Design review of the part built by this model. Coordinates are the model's own, in mm. A direction names the side the tool comes from. Give positions to 0.01 mm unless a question says otherwise; leave off trailing zeros. Write each loop counter-clockwise with the first axis right and the second up, starting at its lowest first coordinate (ties: lowest second). Pieces come first, ordered by that corner, then holes. Notation, with made-up numbers: M 79,47.5 L 138,47.5 A29 cw 138,77.5 Z; hole C 87,-15 d9. An arc over 180 degrees is marked long. Use one line per item in the form item = value. Start each with the question number.
from build123d import *

# Parameters (mm, degrees)
SKETCH1_R           = 215
PLATE_DEPTH         = 20
SKETCH2_R           = 204
SKETCH2_R_2         = 144
COMB_GROOVE_DEPTH   = 4
SKETCH3_R           = 2.75
ROD_HOLES_DEPTH     = 20
SKETCH4_R           = 5
NUT_POCKETS_DEPTH   = 6
SKETCH5_W           = 40
SKETCH5_H           = 30
PD_POCKET_DEPTH     = 8
SKETCH6_W           = 60
SKETCH6_H           = 12
CABLE_CHANNEL_DEPTH = 8


with BuildPart() as part:
    # Sketch1 → Plate (new body)
    with BuildSketch(Plane.XY):
        Circle(SKETCH1_R)
    extrude(amount=PLATE_DEPTH)

    # Sketch2 → Comb_groove (cut)
    with BuildSketch(Plane.XY.offset(16)):
        Circle(SKETCH2_R)
        Circle(SKETCH2_R_2, mode=Mode.SUBTRACT)
    extrude(amount=COMB_GROOVE_DEPTH, mode=Mode.SUBTRACT)

    # Sketch3 → Rod_holes (cut)
    with BuildSketch(Plane.XY):
        with Locations((198.770811906, 64.584551824)):
            Circle(SKETCH3_R)
        with Locations((0, 209)):
            Circle(SKETCH3_R)
        with Locations((-198.770811906, 64.584551824)):
            Circle(SKETCH3_R)
        with Locations((-122.847117729, -169.084551824)):
            Circle(SKETCH3_R)
        with Locations((122.847117729, -169.084551824)):
            Circle(SKETCH3_R)
    extrude(amount=ROD_HOLES_DEPTH, mode=Mode.SUBTRACT)

    # Sketch4 → Nut_pockets (cut)
    with BuildSketch(Plane.XY):
        with Locations((198.770811906, 64.584551824)):
            Circle(SKETCH4_R)
        with Locations((0, 209)):
            Circle(SKETCH4_R)
        with Locations((-198.770811906, 64.584551824)):
            Circle(SKETCH4_R)
        with Locations((-122.847117729, -169.084551824)):
            Circle(SKETCH4_R)
        with Locations((122.847117729, -169.084551824)):
            Circle(SKETCH4_R)
    extrude(amount=NUT_POCKETS_DEPTH, mode=Mode.SUBTRACT)

    # Sketch5 → PD_pocket (cut)
    with BuildSketch(Plane.XY):
        with Locations((145, 0)):
            Rectangle(SKETCH5_W, SKETCH5_H)
    extrude(amount=PD_POCKET_DEPTH, mode=Mode.SUBTRACT)

    # Sketch6 → Cable_channel (cut)
    with BuildSketch(Plane.XY):
        with Locations((190, 0)):
            Rectangle(SKETCH6_W, SKETCH6_H)
    extrude(amount=CABLE_CHANNEL_DEPTH, mode=Mode.SUBTRACT)


solid = part.part
1. To check wall thickness, follow L1, parallel to Y at x = -6.5, z = 17; L2, parallel to Z at x = -102, y = 117.5; L3, parallel to Y at x = -75, z = 16.25. State the ranges of each line that lie inside material, in increasing order.
2. We need section A-A (y = 0). State the section outline as (x, z) points.
3. For faces 1 (the flat face through (-3, 3, 0)), 2 (the cylindrical face through (-18.746, 142.775, 17.972)), 3 (the flat face through (125, -171.2, 6)), list the 3-axis set-ups (+Z, -Z, +X, -X, +Y, -Y) from which the entire face can be reached by the end or side of a thin tool; tool diameter is ignored.
4. Draft analysis for pull direction X (two halves, no side actions). For faces 4 (the flat face through (79, -190, 20)), 5 (the cylindrical face through (-170.62, -130.82, 9.86)), 6 (the flat face through (2.2, 206.8, 6)), state which applies: pulls with the +X half, pulls with the -X half, needs draft (parallel to the pull), parting line crosses it, or undercut.
5. Clearance check with flat-ended pins moving along their axes: pin 1 Ø16 at (x, y) = (-122.85, -169.08) entering from +Z; pin 2 Ø12 at (x, z) = (67.5, 10) entering from +Y; pin 3 Ø10 at (y, z) = (115, 17.5) entering from -X; pin 4 Ø5 at (y, z) = (104.5, 4) entering from +X. State where each tip first meets the part, or that it passes through.
6. We need section D-D (y = 104). State the section outline as (x, z) points, and give its area (3 significant figures).
7. We need section B-B (x = -18). State the section outline as (y, z) points, and give its area (3 significant figures).
8. We need section C-C (z = 13). State the section outline as (x, y) points, and give its area (3 significant figures).
Answer block:
q1.L1 = -214.9 to -203.9, -143.85 to 143.85, 203.9 to 214.9
q1.L2 = 0 to 16
q1.L3 = -201.49 to -189.71, -122.93 to 122.93, 189.71 to 201.49
q2.outline = M -215,0 L 125,0 L 125,8 L 215,8 L 215,20 L 204,20 L 204,16 L 144,16 L 144,20 L -144,20 L -144,16 L -204,16 L -204,20 L -215,20 Z
q3.face_1 = -Z, +X, -X, +Y, -Y
q3.face_2 = +Z
q3.face_3 = -Z
q4.face_4 = needs draft
q4.face_5 = parting line crosses it
q4.face_6 = undercut
q5.pin_1 = 20
q5.pin_2 = 206.02
q5.pin_3 = -184.73
q5.pin_4 = 189.26
q6.outline = M -188.17,0 L 188.17,0 L 188.17,20 L 175.5,20 L 175.5,16 L 99.6,16 L 99.6,20 L -99.6,20 L -99.6,16 L -175.5,16 L -175.5,20 L -188.17,20 Z
q6.area = 6,920 mm^2
q7.outline = M -214.25,0 L 214.25,0 L 214.25,20 L 203.2,20 L 203.2,16 L 142.87,16 L 142.87,20 L -142.87,20 L -142.87,16 L -203.2,16 L -203.2,20 L -214.25,20 Z
q7.area = 8,090 mm^2
q8.outline = C 0,0 d430; hole C -198.77,64.58 d5.5; hole C -122.85,-169.08 d5.5; hole C 0,209 d5.5; hole C 122.85,-169.08 d5.5; hole C 198.77,64.58 d5.5
q8.area = 145,000 mm^2
